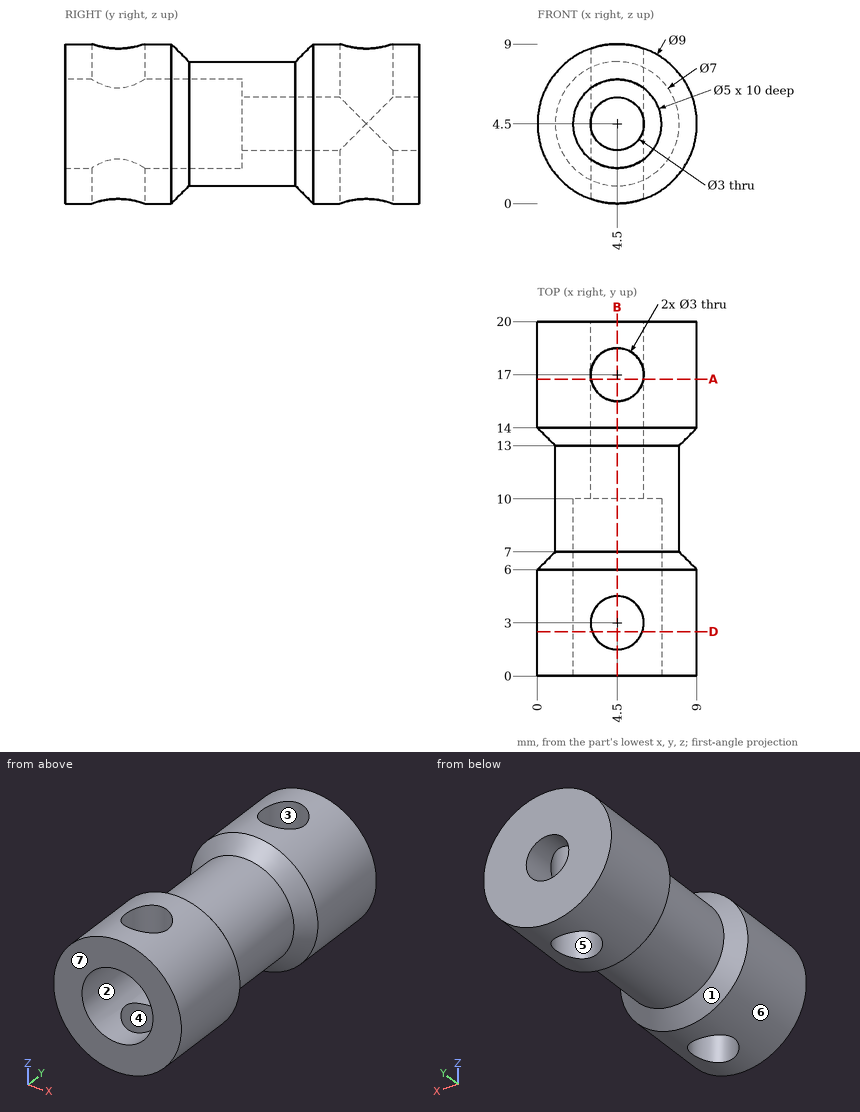
Print and shaded views of the part. All mm, measured from the part's lowest x, y and z. A direction names the side the tool comes from. Give positions to 0.01 mm unless a question says otherwise; leave off trailing zeros. Write each loop counter-clockwise with the first axis right and the second up, starting at its lowest first coordinate (ties: lowest second). Pieces come first, ordered by that corner, then holes. Notation, with made-up numbers: (-5, 35.5) - (5, 35.5) arc R12 cw to (5, 45.5) - close; hole circle Ø3 at (-6, -21). An arc over 180 degrees is marked (long way). One line per question, with ' | ' between items. Start each with the question number.
(1) Slice it at A-A on y = 16.75. Write the cut outline in (x, z).
(2) 3-axis set-ups, long thin cutter, end or side, ignore diameter. For the marked faces 1, 2 and 3: which of +Z, -Z, +X, -X, +Y, -Y reach the whole face in a straight line?
(3) Slice it at B-B on x = 4.5. Give the number of separate pieces and of enclosed holes in the cut face, plus the area to 3 significant figures.
(4) Two-plate mould, pull along X, no slides. Class the marked faces 4, 5, 6 and 7: +X half, -X half, draft (parallel to the pull), parting line (faces both ways), or undercut.
(5) Wall check: line 1 along X through (y, z) = (5, 4.5); line 2 along Y through (x, z) = (3.5, 7); line 3 along X through (y, z) = (15.25, 4.5). Give the ranges that are in metal, low to high. Write a range as from..to.
(6) Pin check, flat tips, straight feed: P1, Ø1, axis at y = 13, z = 7.5, coming from the +X side; P2, Ø1, axis at x = 3.5, y = 9.5, coming from the +Z side; P3, Ø3, axis at x = 3.5, y = 12, coming from the -Z side; P4, Ø2.5, axis at x = 4.5, y = 17, coming from the +Z side. Stop position of each tip, or through.
(7) Slice it at D-D on y = 2.5. Write the cut outline in (x, z), plus the area to 3 significant figures.
Results below:
1) outline: (3.02, 0.25) - (3.02, 4.25) arc R1.5 cw to (3.02, 4.75) - (3.02, 8.75) arc R4.5 ccw to start; (5.98, 0.25) arc R4.5 ccw to (5.98, 8.75) - (5.98, 4.75) arc R1.5 cw to (5.98, 4.25) - close
2) face 1: none | face 2: -Y | face 3: +Z, -Z
3) separate pieces: 6 | enclosed holes: 0 | area: 56.0 mm^2
4) face 4: undercut | face 5: undercut | face 6: parting line | face 7: draft
5) line 1: 0..2, 7..9 | line 2: 0..1.88, 4.12..15.88, 18.12..20 | line 3: 0..3, 6..9
6) P1: x = 7.31 | P2: z = 7.96 | P3: z = 0.59 | P4: through
7) outline: (3.09, 0.23) - (3.09, 2.44) arc R2.5 cw to (3.09, 6.56) - (3.09, 8.77) arc R4.5 ccw to start; (5.91, 0.23) arc R4.5 ccw to (5.91, 8.77) - (5.91, 6.56) arc R2.5 cw to (5.91, 2.44) - close | area: 32.3 mm^2
